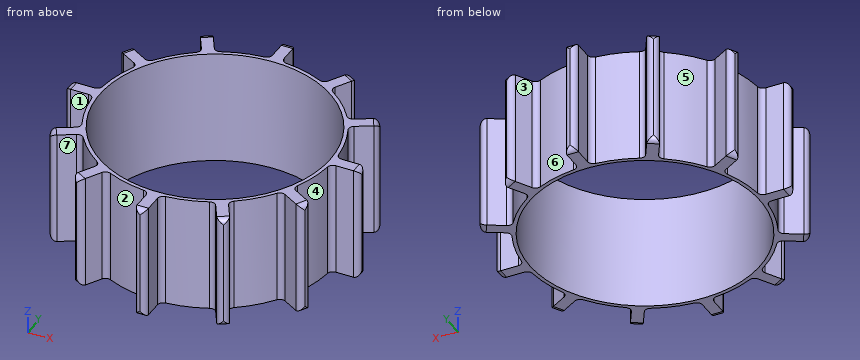
```python
from build123d import *

# Parameters (mm, degrees)
SKIZZE1_R                       = 20
AUFSATZ_LINEAR_AUSTRAGEN2_DEPTH = 20
VERRUNDUNG1_R                   = 1


with BuildPart() as part:
    # Skizze1 → Aufsatz-Linear austragen2 (new body)
    with BuildSketch(Plane.XY):
        with BuildLine():
            Line((-22.692570161, 11.946860953), (-18.362443142, 9.446860953))
            ThreePointArc((-18.362443142, 9.446860953), (-19.946368313, 5.344613281), (-20.625772713, 1))
            Line((-20.625772713, 1), (-25.625772713, 1))
            Line((-25.625772713, 1), (-25.625772713, -1))
            Line((-25.625772713, -1), (-20.625772713, -1))
            ThreePointArc((-20.625772713, -1), (-19.946368313, -5.344613281), (-18.362443142, -9.446860953))
            Line((-18.362443142, -9.446860953), (-22.692570161, -11.946860953))
            Line((-22.692570161, -11.946860953), (-21.692570161, -13.67891176))
            Line((-21.692570161, -13.67891176), (-17.362443142, -11.17891176))
            ThreePointArc((-17.362443142, -11.17891176), (-14.601755032, -14.601755032), (-11.17891176, -17.362443142))
            Line((-11.17891176, -17.362443142), (-13.67891176, -21.692570161))
            Line((-13.67891176, -21.692570161), (-11.946860953, -22.692570161))
            Line((-11.946860953, -22.692570161), (-9.446860953, -18.362443142))
            ThreePointArc((-9.446860953, -18.362443142), (-5.344613281, -19.946368313), (-1, -20.625772713))
            Line((-1, -20.625772713), (-1, -25.625772713))
            Line((-1, -25.625772713), (1, -25.625772713))
            Line((1, -25.625772713), (1, -20.625772713))
            ThreePointArc((1, -20.625772713), (5.344613281, -19.946368313), (9.446860953, -18.362443142))
            Line((9.446860953, -18.362443142), (11.946860953, -22.692570161))
            Line((11.946860953, -22.692570161), (13.67891176, -21.692570161))
            Line((13.67891176, -21.692570161), (11.17891176, -17.362443142))
            ThreePointArc((11.17891176, -17.362443142), (14.601755032, -14.601755032), (17.362443142, -11.17891176))
            Line((17.362443142, -11.17891176), (21.692570161, -13.67891176))
            Line((21.692570161, -13.67891176), (22.692570161, -11.946860953))
            Line((22.692570161, -11.946860953), (18.362443142, -9.446860953))
            ThreePointArc((18.362443142, -9.446860953), (19.946368313, -5.344613281), (20.625772713, -1))
            Line((20.625772713, -1), (25.625772713, -1))
            Line((25.625772713, -1), (25.625772713, 1))
            Line((25.625772713, 1), (20.625772713, 1))
            ThreePointArc((20.625772713, 1), (19.946368313, 5.344613281), (18.362443142, 9.446860953))
            Line((18.362443142, 9.446860953), (22.692570161, 11.946860953))
            Line((22.692570161, 11.946860953), (21.692570161, 13.67891176))
            Line((21.692570161, 13.67891176), (17.362443142, 11.17891176))
            ThreePointArc((17.362443142, 11.17891176), (14.601755032, 14.601755032), (11.17891176, 17.362443142))
            Line((11.17891176, 17.362443142), (13.67891176, 21.692570161))
            Line((13.67891176, 21.692570161), (11.946860953, 22.692570161))
            Line((11.946860953, 22.692570161), (9.446860953, 18.362443142))
            ThreePointArc((9.446860953, 18.362443142), (5.344613281, 19.946368313), (1, 20.625772713))
            Line((1, 20.625772713), (1, 25.625772713))
            Line((1, 25.625772713), (-1, 25.625772713))
            Line((-1, 25.625772713), (-1, 20.625772713))
            ThreePointArc((-1, 20.625772713), (-5.344613281, 19.946368313), (-9.446860953, 18.362443142))
            Line((-9.446860953, 18.362443142), (-11.946860953, 22.692570161))
            Line((-11.946860953, 22.692570161), (-13.67891176, 21.692570161))
            Line((-13.67891176, 21.692570161), (-11.17891176, 17.362443142))
            ThreePointArc((-11.17891176, 17.362443142), (-14.601755032, 14.601755032), (-17.362443142, 11.17891176))
            Line((-17.362443142, 11.17891176), (-21.692570161, 13.67891176))
            Line((-21.692570161, 13.67891176), (-22.692570161, 11.946860953))
        make_face()
        Circle(SKIZZE1_R, mode=Mode.SUBTRACT)
    extrude(amount=AUFSATZ_LINEAR_AUSTRAGEN2_DEPTH)

    # Verrundung1
    verrundung1_edges = [part.edges().sort_by_distance(p)[0] for p in [
        (25.625772713, 0, 20),
        (22.192570161, 12.812886356, 20),
        (-25.625772713, 0, 20),
        (12.812886356, 22.192570161, 20),
        (0, 25.625772713, 20),
        (-12.812886356, 22.192570161, 20),
        (-22.192570161, 12.812886356, 20),
        (-22.192570161, -12.812886356, 20),
        (-12.812886356, -22.192570161, 20),
        (-22.192570161, 12.812886356, 0),
        (-12.812886356, 22.192570161, 0),
        (0, 25.625772713, 0),
        (12.812886356, 22.192570161, 0),
        (22.192570161, 12.812886356, 0),
        (25.625772713, 0, 0),
        (22.192570161, -12.812886356, 0),
        (12.812886356, -22.192570161, 0),
        (0, -25.625772713, 0),
        (-12.812886356, -22.192570161, 0),
        (0, -25.625772713, 20),
        (-22.192570161, -12.812886356, 0),
        (-25.625772713, 0, 0),
        (12.812886356, -22.192570161, 20),
        (-18.362443142, 9.446860953, 10),
        (-22.692570161, 11.946860953, 10),
        (-21.692570161, 13.67891176, 10),
        (-17.362443142, 11.17891176, 10),
        (-11.17891176, 17.362443142, 10),
        (-13.67891176, 21.692570161, 10),
        (-11.946860953, 22.692570161, 10),
        (-9.446860953, 18.362443142, 10),
        (-1, 20.625772713, 10),
        (-1, 25.625772713, 10),
        (1, 25.625772713, 10),
        (1, 20.625772713, 10),
        (9.446860953, 18.362443142, 10),
        (11.946860953, 22.692570161, 10),
        (13.67891176, 21.692570161, 10),
        (11.17891176, 17.362443142, 10),
        (17.362443142, 11.17891176, 10),
        (21.692570161, 13.67891176, 10),
        (22.692570161, 11.946860953, 10),
        (18.362443142, 9.446860953, 10),
        (20.625772713, 1, 10),
        (25.625772713, 1, 10),
        (25.625772713, -1, 10),
        (20.625772713, -1, 10),
        (18.362443142, -9.446860953, 10),
        (22.692570161, -11.946860953, 10),
        (21.692570161, -13.67891176, 10),
        (17.362443142, -11.17891176, 10),
        (11.17891176, -17.362443142, 10),
        (13.67891176, -21.692570161, 10),
        (11.946860953, -22.692570161, 10),
        (9.446860953, -18.362443142, 10),
        (1, -20.625772713, 10),
        (1, -25.625772713, 10),
        (-1, -25.625772713, 10),
        (-1, -20.625772713, 10),
        (-9.446860953, -18.362443142, 10),
        (-11.946860953, -22.692570161, 10),
        (-13.67891176, -21.692570161, 10),
        (-11.17891176, -17.362443142, 10),
        (-17.362443142, -11.17891176, 10),
        (-21.692570161, -13.67891176, 10),
        (-22.692570161, -11.946860953, 10),
        (-18.362443142, -9.446860953, 10),
        (-20.625772713, -1, 10),
        (-25.625772713, -1, 10),
        (-25.625772713, 1, 10),
        (-20.625772713, 1, 10),
        (22.192570161, -12.812886356, 20),
    ]]
    fillet(verrundung1_edges, radius=VERRUNDUNG1_R - 0.0001)  # a hair under: the kernel refuses the full size


solid = part.part
```
Check sheet for the modelled part. Datum: model origin and axes. Units: mm. Face numbers are marked on the shaded views. A direction names the side the tool comes from. Round coordinates to 2 decimals unless told otherwise and drop trailing zeros. Order: outer loops, then holes, each group sorted by start corner. A loop starts at its lowest first (then second) coordinate and runs counter-clockwise, first axis right, second up. Notation, with made-up numbers: (42, 68) - (89, 68) arc R38 cw to (89, 107) - close; hole circle Ø1 at (76, 47.5). An arc over 180 degrees is marked (long way). Answer as CSV lines item,"result". Start each with the question number.
1) Tool access check on the marked faces 1, 2, 3 and 4. Record the directions out of +Z, -Z, +X, -X, +Y, -Y that give a thin tool (end or side, any length) a straight path to the whole face; none if there is none.
2) Section check B-B (y = -14.5). Record the cut outline in (x, z).
3) Draft check along Y on the marked faces 5, 6 and 7. Enter one of: +Y half, -Y half, draft (parallel to the pull), parting line (faces both ways), or undercut.
4) Section check A-A (y = 4). Record the cut outline in (x, z).
5) Depth check by flat-ended pin: pin 1 (0.9 mm diameter, centred on x = 24, z = 10, fed in from +Y); pin 2 (3.5 mm diameter, centred on y = 23.5, z = 8, fed in from +X); pin 3 (4 mm diameter, centred on y = 7.5, z = 15.5, fed in from -X). Enter the tip coordinate at first touch or a pass-through.
6) Scan lines: probe 1 along Y at (x, z) = (0, 8); probe 2 along Y at (x, z) = (21, 4); probe 3 along Y at (x, z) = (3, 19.25). Record each from-to range of solid material in increasing order.
Determined:
1,face 1,"+Z, -Z, -X"
1,face 2,"+Z, -Z, -Y"
1,face 3,"+Z, -Z, +Y"
1,face 4,"+Z, -Z, +X"
2,outline,"(-14.7, 0) - (-13.77, 0) - (-13.77, 20) - (-14.7, 20) - close; (13.77, 0) - (14.7, 0) - (14.7, 20) - (13.77, 20) - close"
3,face 5,"undercut"
3,face 6,"+Y half"
3,face 7,"-Y half"
4,outline,"(-20.26, 0) - (-19.6, 0) - (-19.6, 20) - (-20.26, 20) - close; (19.6, 0) - (20.26, 0) - (20.26, 20) - (19.6, 20) - close"
5,pin 1,"y = 1"
5,pin 2,"x = 13.22"
5,pin 3,"x = -19.9"
6,probe 1,"-25.63 to -20, 20 to 25.63"
6,probe 2,"-13.26 to -10.97, -1.17 to 1.17, 10.97 to 13.26"
6,probe 3,"-20.43 to -19.77, 19.77 to 20.43"
